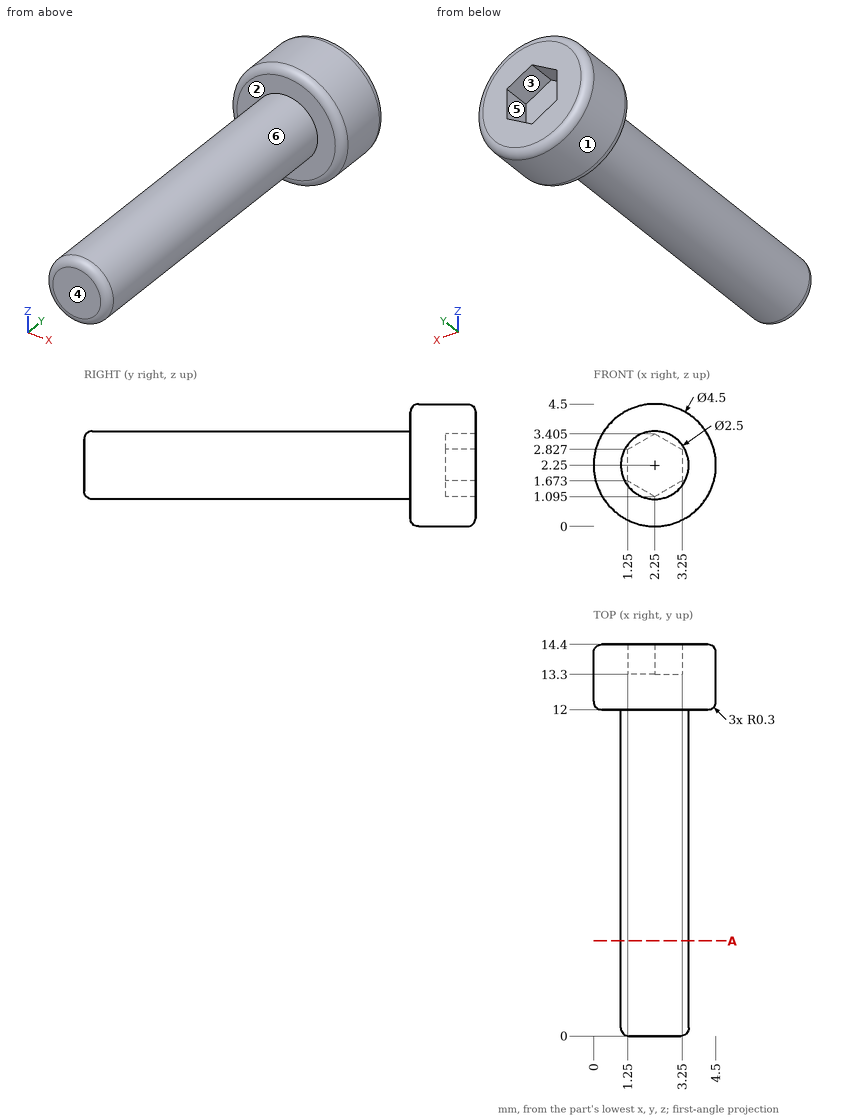
Geometry check sheet. Reference: drawing and pictorial views, mm from the part's lowest x, y, z. A direction names the side the tool comes from. Coordinates: 2 decimals unless noted, no trailing zeros. Order: outer loops, then holes, each group sorted by start corner. A loop starts at its lowest first (then second) coordinate and runs counter-clockwise, first axis right, second up. Notation, with made-up numbers: (15.5, 74) - (53.5, 74) arc R8 cw to (53.5, 87) - close; hole circle Ø11 at (31, 65). An arc over 180 degrees is marked (long way). One line per item, written item: value.
(1) Release check for a two-part mould opening along X. For the marked faces 4, 5 and 6 record: +X half, -X half, draft (parallel to the pull), parting line (faces both ways), or undercut.
Data:
face 4: draft
face 5: undercut
face 6: parting line
(2) Access from +Z, -Z, +X, -X, +Y, -Y to the whole of each face (thin tool, end or side, straight path). Record for the marked faces 1, 2 and 3.
Data:
face 1: +Y, -Y
face 2: -Y
face 3: +Y
(3) Thickness scan on probe 1 along Y at (x, z) = (2.4, 3.65); probe 2 along Z at (x, y) = (2.2, 1.25); probe 3 along Y at (x, z) = (2, 2). Record the ranges inside material, lowest first. Write a range as from..to.
Data:
probe 1: y = 12..14.4
probe 2: z = 1..3.5
probe 3: y = 0..13.3
(4) Sectioned sample at A-A (y = 3.5). Enter the section's corners in (x, z).
Data:
outline: circle Ø2.5 at (2.25, 2.25)
